from build123d import *

# Parameters (mm, degrees)
SCHIZZO1_W                   = 150
SCHIZZO1_H                   = 60
ESTRUSIONE_ESTRUSIONE1_DEPTH = 38
SVUOTA1_T                    = -4
SCHIZZO2_R                   = 1.75
TAGLIO_ESTRUSIONE1_DEPTH     = 10
SCHIZZO4_R                   = 1.75
TAGLIO_ESTRUSIONE2_DEPTH     = 10
RIPETIZIONE_A_L1_COUNT       = 2
RIPETIZIONE_A_L1_PITCH       = 15
RIPETIZIONE_A_L1_COUNT_DIR2  = 2
RIPETIZIONE_A_L1_PITCH_DIR2  = 20
TAGLIO_ESTRUSIONE3_DEPTH     = 10
RIPETIZIONE_A_L2_COUNT       = 4
RIPETIZIONE_A_L2_PITCH       = 14.666666667
SCHIZZO6_W                   = 14.123548546
SCHIZZO6_H                   = 8
TAGLIO_ESTRUSIONE4_DEPTH     = 10
SPECCHIA2_COPY_1_SKETCH_W    = 14.123548546
SPECCHIA2_COPY_1_SKETCH_H    = 8
SPECCHIA2_COPY_1_DEPTH       = 10
SPECCHIA2_COPY_2_DEPTH       = 10
SPECCHIA2_COPY_3_DEPTH       = 10
SPECCHIA2_COPY_4_DEPTH       = 10
SPECCHIA2_COPY_5_DEPTH       = 10
ESTRUSIONE_ESTRUSIONE3_DEPTH = 4.5
RACCORDO3_R                  = 2


with BuildPart() as part:
    # Schizzo1 → Estrusione-Estrusione1 (new body, symmetric)
    with BuildSketch(Plane.XY):
        Rectangle(SCHIZZO1_W, SCHIZZO1_H)
    extrude(amount=ESTRUSIONE_ESTRUSIONE1_DEPTH, both=True)

    # Svuota1
    svuota1_openings = [part.faces().sort_by_distance(p)[0] for p in [
        (0, 0, -38),
    ]]
    offset(amount=SVUOTA1_T, openings=svuota1_openings, kind=Kind.INTERSECTION)

    # Schizzo2 → Taglio-Estrusione1 (cut)
    with BuildSketch(Plane(origin=(0, 0, 34), x_dir=(-1, 0, 0), z_dir=(0, 0, -1))):
        with Locations((20, 0)):
            Circle(SCHIZZO2_R)
    taglio_estrusione1 = extrude(amount=-TAGLIO_ESTRUSIONE1_DEPTH, mode=Mode.SUBTRACT)

    # Specchia1: Taglio-Estrusione1 across plane
    add(taglio_estrusione1.mirror(Plane(origin=(0, 0, 0), x_dir=(0, 0, 1), z_dir=(1, 0, 0))), mode=Mode.SUBTRACT)

    # Schizzo4 → Taglio-Estrusione2 (cut)
    with BuildSketch(Plane(origin=(0, 30, 0), x_dir=(1, 0, 0), z_dir=(0, 1, 0))):
        with Locations((10, 7.5)):
            Circle(SCHIZZO4_R)
    taglio_estrusione2 = extrude(amount=-TAGLIO_ESTRUSIONE2_DEPTH, mode=Mode.SUBTRACT)

    # Ripetizione a L1: Taglio-Estrusione2 2 × 2
    with Locations(*[(-j * RIPETIZIONE_A_L1_PITCH_DIR2, 0, i * RIPETIZIONE_A_L1_PITCH) for i in range(RIPETIZIONE_A_L1_COUNT) for j in range(RIPETIZIONE_A_L1_COUNT_DIR2) if (i, j) != (0, 0)]):
        add(taglio_estrusione2, mode=Mode.SUBTRACT)

    # Schizzo5 → Taglio-Estrusione3 (cut)
    with BuildSketch(Plane.ZY.offset(75)):
        with BuildLine():
            Line((-25, 26), (25, 26))
            ThreePointArc((25, 26), (29, 22), (25, 18))
            Line((25, 18), (-25, 18))
            ThreePointArc((-25, 18), (-29, 22), (-25, 26))
        make_face()
    taglio_estrusione3 = extrude(amount=-TAGLIO_ESTRUSIONE3_DEPTH, mode=Mode.SUBTRACT)

    # Ripetizione a L2: Taglio-Estrusione3 ×4
    with Locations(*[(0, -i * RIPETIZIONE_A_L2_PITCH, 0) for i in range(1, RIPETIZIONE_A_L2_COUNT)]):
        add(taglio_estrusione3, mode=Mode.SUBTRACT)

    # Schizzo6 → Taglio-Estrusione4 (cut)
    with BuildSketch(Plane.ZY.offset(75)):
        with Locations((-30.938225727, -22)):
            Rectangle(SCHIZZO6_W, SCHIZZO6_H)
    taglio_estrusione4 = extrude(amount=-TAGLIO_ESTRUSIONE4_DEPTH, mode=Mode.SUBTRACT)

    # Specchia3: Taglio-Estrusione4 across plane
    add(taglio_estrusione4.mirror(Plane.ZX), mode=Mode.SUBTRACT)

    # Specchia2: Taglio-Estrusione4 across plane
    add(taglio_estrusione4.mirror(Plane(origin=(0, 0, 0), x_dir=(0, 0, 1), z_dir=(1, 0, 0))), mode=Mode.SUBTRACT)

    # Specchia2 copy 1 sketch → Specchia2 copy 1 (cut)
    with BuildSketch(Plane(origin=(75, 0, 0), x_dir=(0, 0, 1), z_dir=(1, 0, 0))):
        with Locations((-30.938225727, -22)):
            Rectangle(SPECCHIA2_COPY_1_SKETCH_W, SPECCHIA2_COPY_1_SKETCH_H)
    extrude(amount=-SPECCHIA2_COPY_1_DEPTH, mode=Mode.SUBTRACT)

    # Specchia2 copy 2 sketch → Specchia2 copy 2 (cut)
    with BuildSketch(Plane(origin=(75, -14.666666667, 0), x_dir=(0, 0, 1), z_dir=(1, 0, 0))):
        with BuildLine():
            Line((-25, -26), (25, -26))
            ThreePointArc((25, -26), (29, -22), (25, -18))
            Line((25, -18), (-25, -18))
            ThreePointArc((-25, -18), (-29, -22), (-25, -26))
        make_face()
    extrude(amount=-SPECCHIA2_COPY_2_DEPTH, mode=Mode.SUBTRACT)

    # Specchia2 copy 3 sketch → Specchia2 copy 3 (cut)
    with BuildSketch(Plane(origin=(75, -29.333333333, 0), x_dir=(0, 0, 1), z_dir=(1, 0, 0))):
        with BuildLine():
            Line((-25, -26), (25, -26))
            ThreePointArc((25, -26), (29, -22), (25, -18))
            Line((25, -18), (-25, -18))
            ThreePointArc((-25, -18), (-29, -22), (-25, -26))
        make_face()
    extrude(amount=-SPECCHIA2_COPY_3_DEPTH, mode=Mode.SUBTRACT)

    # Specchia2 copy 4 sketch → Specchia2 copy 4 (cut)
    with BuildSketch(Plane(origin=(75, -44, 0), x_dir=(0, 0, 1), z_dir=(1, 0, 0))):
        with BuildLine():
            Line((-25, -26), (25, -26))
            ThreePointArc((25, -26), (29, -22), (25, -18))
            Line((25, -18), (-25, -18))
            ThreePointArc((-25, -18), (-29, -22), (-25, -26))
        make_face()
    extrude(amount=-SPECCHIA2_COPY_4_DEPTH, mode=Mode.SUBTRACT)

    # Specchia2 copy 5 sketch → Specchia2 copy 5 (cut)
    with BuildSketch(Plane(origin=(75, 0, 0), x_dir=(0, 0, 1), z_dir=(1, 0, 0))):
        with BuildLine():
            Line((-25, -26), (25, -26))
            ThreePointArc((25, -26), (29, -22), (25, -18))
            Line((25, -18), (-25, -18))
            ThreePointArc((-25, -18), (-29, -22), (-25, -26))
        make_face()
    extrude(amount=-SPECCHIA2_COPY_5_DEPTH, mode=Mode.SUBTRACT)

    # Schizzo9 → Estrusione-Estrusione3 (add, symmetric)
    with BuildSketch(Plane(origin=(0, 0, 0), x_dir=(1, 0, 0), z_dir=(0, 1, 0))):
        Polygon((-75, 30.2), (-75.5, 30.2), (-75, 32.2), align=None)
    estrusione_estrusione3 = extrude(amount=ESTRUSIONE_ESTRUSIONE3_DEPTH, both=True)

    # Specchia11: Estrusione-Estrusione3 across plane
    add(estrusione_estrusione3.mirror(Plane(origin=(0, 0, 0), x_dir=(0, 0, 1), z_dir=(1, 0, 0))))

    # Raccordo3
    raccordo3_edges = [part.edges().sort_by_distance(p)[0] for p in [
        (75, -30, 0),
        (-75, -30, 0),
        (-75, 30, 0),
        (75, 30, 0),
    ]]
    fillet(raccordo3_edges, radius=RACCORDO3_R)


solid = part.part
Model file for the job. Use its own axes, mm. A direction names the side the tool comes from. Give positions to 0.01 mm unless a question says otherwise; leave off trailing zeros. Order: outer loops, then holes, each group sorted by start corner. A loop starts at its lowest first (then second) coordinate and runs counter-clockwise, first axis right, second up. Notation, with made-up numbers: M -31,4.5 L 25,4.5 A29 ccw 25,41.5 Z; hole C 0,23.25 d1. An arc over 180 degrees is marked long. Put each result on its own line as item: value. Start each with the question number.
(1) Pull direction Y, two halves, no side cores. Call faces 1 (the face through (-1, -28, -38)), 2 (the face through (-73, 3.333, 0)): released by +Y, released by -Y, zero draft, split by the parting line, or undercut.
(2) Band-saw the part on D-D on x = 51. Give the cut face in (y, z).
(3) Band-saw the part on C-C on y = -9. Give the cut face in (x, z), then the cut area to 3 significant figures.
(4) Band-saw the part on A-A on x = 10. Give the cut face in (y, z).
(5) Tool access for faces 3 (the face through (-71, 0, -1)), 4 (the face through (73, 11.333, 0)), 5 (the face through (73, -18, -7)), 6 (the face through (-1, 28, -38)): list every direction of +Z, -Z, +X, -X, +Y, -Y with a clear straight run to the whole face (end or side of a thin tool).
(6) Drill centre lines: L1, parallel to Z at x = -10, y = 28; L2, parallel to X at y = 28.3, z = 7.5; L3, parallel to X at y = 2, z = -15. Where is each one in solid material? Low to high. Write a range as [from, to].
(7) Band-saw the part on B-B on y = 22. Give the cut face in (x, z), then the cut area to 3 significant figures.
(8) Pin check, flat tips, straight feed: pin 1 Ø2 at (x, z) = (10, 7.5) entering from +Y; pin 2 Ø12 at (x, y) = (-41, -6) entering from -Z; pin 3 Ø1.2 at (x, z) = (74, 4) entering from +Y; pin 4 Ø1.5 at (y, z) = (19, 4) entering from +X. Stop position of each tip, or through.
Results below:
1. face 1: zero draft
1. face 2: undercut
2. outline: M -30,-38 L -26,-38 L -26,34 L 26,34 L 26,-38 L 30,-38 L 30,38 L -30,38 Z
3. outline: M -75,-38 L -71,-38 L -71,-28.64 L -75,-28.64 Z; M -75,28.64 L -71,28.64 L -71,34 L 71,34 L 71,28.64 L 75,28.64 L 75,38 L -75,38 Z; M 71,-38 L 75,-38 L 75,-28.64 L 71,-28.64 Z
3. area: 718 mm2
4. outline: M -30,-38 L -26,-38 L -26,34 L 26,34 L 26,9.25 L 30,9.25 L 30,38 L -30,38 Z; M 26,-38 L 30,-38 L 30,-9.25 L 26,-9.25 Z; M 26,-5.75 L 30,-5.75 L 30,5.75 L 26,5.75 Z
5. face 3: -Z
5. face 4: +X, -X
5. face 5: -Z, +X, -X
5. face 6: -Z, +X, -X, +Y, -Y
6. L1: z = [-38, -9.25], [-5.75, 5.75], [9.25, 38]
6. L2: x = [-74.98, -11.75], [-8.25, 8.25], [11.75, 74.98]
6. L3: x = [-75, -71], [71, 75]
7. outline: M -75,29 L -71,29 L -71,34 L 71,34 L 71,29 L 75,29 L 75,38 L -75,38 Z
7. area: 640 mm2
8. pin 1: stops at y = -26
8. pin 2: stops at z = 34
8. pin 3: stops at y = 29.96
8. pin 4: passes through
